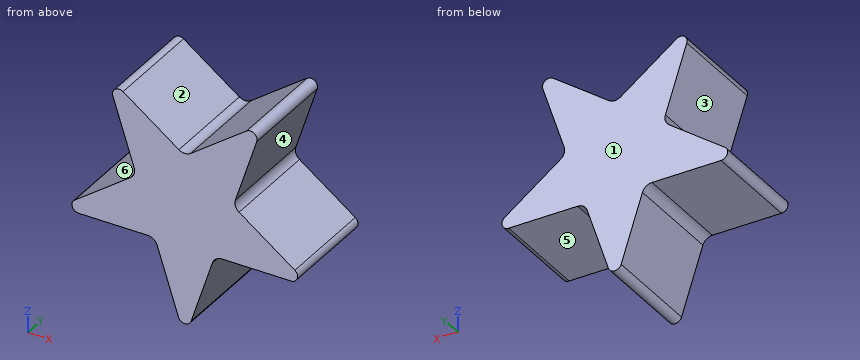
```python
from build123d import *

# Parameters (mm, degrees)
BOSS_EXTRUDE1_DEPTH = 30
FILLET1_R           = 2
FILLET2_R           = 3


with BuildPart() as part:
    # Sketch2 → Boss-Extrude1 (new body)
    with BuildSketch(Plane(origin=(0, 0, 0), x_dir=(1, 0, 0), z_dir=(0, 1, 0))):
        Polygon((0, 39.962281052), (-8.9720911, 12.349023979), (-38.0063878, 12.349023979), (-14.51714835, -4.716907432), (-23.48923945, -32.330164505), (0, -15.264233094), (23.48923945, -32.330164505), (14.51714835, -4.716907432), (38.0063878, 12.349023979), (8.9720911, 12.349023979), align=None)
    extrude(amount=BOSS_EXTRUDE1_DEPTH)

    # Fillet1
    fillet1_edges = [part.edges().sort_by_distance(p)[0] for p in [
        (23.48923945, 15, 32.330164505),
        (-23.48923945, 15, 32.330164505),
        (-38.0063878, 15, -12.349023979),
        (0, 15, -39.962281052),
        (38.0063878, 15, -12.349023979),
    ]]
    fillet(fillet1_edges, radius=FILLET1_R)

    # Fillet2
    fillet2_edges = [part.edges().sort_by_distance(p)[0] for p in [
        (14.51714835, 15, 4.716907432),
        (0, 15, 15.264233094),
        (-14.51714835, 15, 4.716907432),
        (-8.9720911, 15, -12.349023979),
        (8.9720911, 15, -12.349023979),
    ]]
    fillet(fillet2_edges, radius=FILLET2_R)


solid = part.part
```
Could you check a few things on this model? Use its own coordinates, in mm. Face numbers are marked on the shaded views. A direction names the side the tool comes from. Coordinates: 2 decimals unless noted, no trailing zeros. Write each loop counter-clockwise with the first axis right and the second up, starting at its lowest first coordinate (ties: lowest second). Pieces come first, ordered by that corner, then holes. Notation, with made-up numbers: (-9, 37.5) -> (26, 37.5) arc R29 cw to (26, 58.5) -> close; hole circle Ø5 at (87, 22.25). An arc over 180 degrees is marked (long way). Return JSON: item names as keys, results as strings.
(1) I need wall thicknesses on L1, parallel to X at y = 25.5, z = 20.5; L2, parallel to X at y = 9.25, z = 24.5; L3, parallel to X at y = 27.25, z = -28. Which ranges of each line are inside material? Lowest first, please.
Numbers:
{"L1": "x = -19.65 to -7.21, 7.21 to 19.65", "L2": "x = -20.95 to -12.71, 12.71 to 20.95", "L3": "x = -3.89 to 3.89"}
(2) Imagine slicing it at B-B, the plane x = 30. Please give me the cut outline in (y, z), then the cut area to 3 significant figures.
Numbers:
{"outline": "(0, -12.35) -> (30, -12.35) -> (30, -6.53) -> (0, -6.53) -> close", "area": "175 mm2"}
(3) Which directions (+Z, -Z, +X, -X, +Y, -Y) give clear straight access to the entire face, cutting with the end or side of a thin tool? Please do the marked faces 4, 5 and 6.
Numbers:
{"face 4": "+X, +Y, -Y", "face 5": "-Z, +X, +Y, -Y", "face 6": "-X, +Y, -Y"}
(4) Imagine slicing it at C-C, the plane z = 1. Please give me the cut outline in (x, y), then the cut area to 3 significant figures.
Numbers:
{"outline": "(-19.63, 0) -> (19.63, 0) -> (19.63, 30) -> (-19.63, 30) -> close", "area": "1,180 mm2"}
(5) We'd pull the mould along X, two halves only. Please class the marked faces 1, 2 and 3: +X half, -X half, draft (parallel to the pull), parting line (faces both ways), or undercut.
Numbers:
{"face 1": "draft", "face 2": "undercut", "face 3": "-X half"}
(6) Imagine slicing it at A-A, the plane y = 13.25. Please give me the cut outline in (x, z).
Numbers:
{"outline": "(-33.03, -8.73) arc R2 ccw to (-31.85, -12.35) -> (-11.15, -12.35) arc R3 cw to (-8.3, -14.42) -> (-1.9, -34.11) arc R2 ccw to (1.9, -34.11) -> (8.3, -14.42) arc R3 cw to (11.15, -12.35) -> (31.85, -12.35) arc R2 ccw to (33.03, -8.73) -> (16.28, 3.44) arc R3 cw to (15.19, 6.79) -> (21.59, 26.48) arc R2 ccw to (18.51, 28.71) -> (1.76, 16.55) arc R3 cw to (-1.76, 16.55) -> (-18.51, 28.71) arc R2 ccw to (-21.59, 26.48) -> (-15.19, 6.79) arc R3 cw to (-16.28, 3.44) -> close"}
(7) I'm going to push flat-ended pins straight in: pin 1 (2 mm diameter, centred on x = -17, y = 27, fed in from -Z); pin 2 (3 mm diameter, centred on y = 22, z = 20.5, fed in from -X); pin 3 (5 mm diameter, centred on y = 24.5, z = 7, fed in from +X). Where does each tip first touch, or does it pass through?
Numbers:
{"pin 1": "stops at z = -12.35", "pin 2": "stops at x = -20.13", "pin 3": "stops at x = 16.07"}
